Autodesk Inventor part; units mm, degrees
ref_plane "YZ Plane" through (0, 0, 0) normal (1, 0, 0) x (0, 1, 0)
ref_plane "XZ Plane" through (0, 0, 0) normal (0, 1, 0) x (-1, 0, 0)
ref_plane "XY Plane" through (0, 0, 0) normal (0, 0, 1) x (1, 0, 0)
sketch "Sketch1" plane through (0, 0, 0) normal (0, 1, 0) x (-1, 0, 0)
  circle A0 centre (0, 0) radius 2.032
  dimension "d0" = 4.064
extrude "Extrusion1" add sketch "Sketch1" along normal blind 19.05
sketch "Sketch2" plane through (0, 0, 0) normal (0, 0, 1) x (1, 0, 0)
  circle A0 centre (0, 29.2638) radius 6.35
  line L0 (2.032, 19.05) -> (-2.032, 19.05)
  circle A1 centre (0, 29.2638) radius 10.414
  point P0 (0, 0)
  dimension "d3" = 4.064
  dimension "d4" = 12.7
extrude "Extrusion2" add sketch "Sketch2" along normal mid plane 4.064 contours L0 A1 picked at (0.2551, 20.3534)
properties part number "EyeBolt"
Check sheet for the modelled part. Datum: model origin and axes. Units: mm. A direction names the side the tool comes from. Coordinates: 2 decimals unless noted, no trailing zeros. Order: outer loops, then holes, each group sorted by start corner. A loop starts at its lowest first (then second) coordinate and runs counter-clockwise, first axis right, second up. Notation, with made-up numbers: (-24, 1) -> (7, 1) arc R23 ccw to (7, 31) -> close; hole circle Ø9 at (-28.5, 44.25). An arc over 180 degrees is marked (long way). Write item = value, one per line. Start each with the question number.
1) Cross-section at B-B (x = 5.75). Enter the section's corners in (y, z), then the cut area to 3 significant figures.
2) Mould release check, pull along Y, two halves, no side actions. Record for faces 1 (the flat face through (-5, 25, -2.032)), 2 (the flat face through (-1.6, 19.05, 1.6)), 3 (the cylindrical face through (-1.38, 35.46, -0.03)): +Y half, -Y half, draft (parallel to the pull), parting line (faces both ways), or undercut.
3) Cross-section at A-A (y = 32). Enter the section's corners in (x, z).
4) Access from +Z, -Z, +X, -X, +Y, -Y to the whole of each face (thin tool, end or side, straight path). Record for faces 4 (the flat face through (1.6, 19.05, -1.5)), 5 (the flat face through (-1.5, 19.05, -1.6)), 6 (the cylindrical face through (0.44, 9.392, 1.984)).
5) Cross-section at D-D (x = -1). Enter the section's corners in (y, z).
6) Go/stop test with a flat-tipped pin: P1, Ø1.5, axis at y = 13.5, z = 1, coming from the +X side. Record where the tip stops, or that it passes through.
7) Material ranges on L1, parallel to Y at x = 0, z = 0.6; L2, parallel to X at y = 15.5, z = 0; L3, parallel to X at y = 34.5, z = 1.25, recorded low to high.
8) Cross-section at C-C (z = 1.3). Enter the section's corners in (x, y), then the cut area to 3 significant figures.
Ans:
q1.outline = (20.58, -2.03) -> (26.57, -2.03) -> (26.57, 2.03) -> (20.58, 2.03) -> close; (31.96, -2.03) -> (37.95, -2.03) -> (37.95, 2.03) -> (31.96, 2.03) -> close
q1.area = 48.7 mm²
q2.face_1 = draft
q2.face_2 = -Y half
q2.face_3 = undercut
q3.outline = (-10.05, -2.03) -> (-5.73, -2.03) -> (-5.73, 2.03) -> (-10.05, 2.03) -> close; (5.73, -2.03) -> (10.05, -2.03) -> (10.05, 2.03) -> (5.73, 2.03) -> close
q4.face_4 = -Z, +X, -Y
q4.face_5 = -Z, -X, -Y
q4.face_6 = -Y
q5.outline = (0, -1.77) -> (19.05, -1.77) -> (19.05, -2.03) -> (22.99, -2.03) -> (22.99, 2.03) -> (19.05, 2.03) -> (19.05, 1.77) -> (0, 1.77) -> close; (35.53, -2.03) -> (39.63, -2.03) -> (39.63, 2.03) -> (35.53, 2.03) -> close
q6.P1 = 2.02
q7.L1 = 0 to 22.91, 35.61 to 39.68
q7.L2 = -2.03 to 2.03
q7.L3 = -9 to -3.59, 3.59 to 9
q8.outline = (-2.03, 19.05) -> (-1.56, 19.05) -> (-1.56, 0) -> (1.56, 0) -> (1.56, 19.05) -> (2.03, 19.05) arc R10.41 ccw (long way) to start; hole circle Ø12.7 at (0, 29.26)
q8.area = 273 mm²
